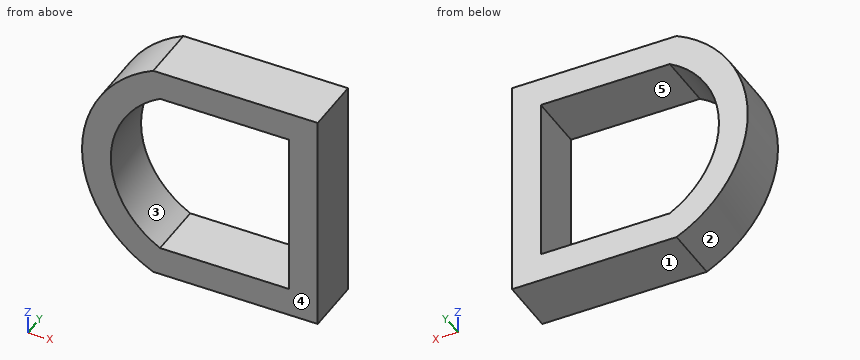
Autodesk Inventor part; units mm, degrees
ref_plane "YZ Plane" through (0, 0, 0) normal (1, 0, 0) x (0, 1, 0)
ref_plane "XZ Plane" through (0, 0, 0) normal (0, 1, 0) x (-1, 0, 0)
ref_plane "XY Plane" through (0, 0, 0) normal (0, 0, 1) x (1, 0, 0)
sketch "Sketch1" plane through (0, 0, 0) normal (0, 1, 0) x (-1, 0, 0)
  line L0 (53.122, 125.6518) -> (38.898, 125.6518)
  line L1 (38.898, 125.6518) -> (38.898, 107.3638)
  line L2 (38.898, 107.3638) -> (53.122, 107.3638)
  arc A0 (53.122, 107.3638) -> (53.122, 125.6518) centre (48.1382, 116.5078) ccw
  line L3 (51.0559, 55.1199) -> (37.0859, 55.1199)
  line L4 (37.0859, 55.1199) -> (37.0859, 37.0859)
  line L5 (37.0859, 37.0859) -> (51.0559, 37.0859)
  arc A1 (51.0559, 37.0859) -> (51.0559, 55.1199) centre (39.6314, 46.1029) ccw
  line L6 (61.7452, 17.3999) -> (47.7752, 17.3999)
  line L7 (47.7752, 17.3999) -> (47.7752, -0.6341)
  line L8 (47.7752, -0.6341) -> (61.7452, -0.6341)
  arc A2 (61.7452, -0.6341) -> (61.7452, 17.3999) centre (49.459, 8.3829) ccw
  line L9 (89.1373, 73.7746) -> (75.1673, 73.7746)
  line L10 (75.1673, 73.7746) -> (75.1673, 55.7406)
  line L11 (75.1673, 55.7406) -> (89.1373, 55.7406)
  arc A3 (89.1373, 55.7406) -> (89.1373, 73.7746) centre (83.9272, 64.7576) ccw
  line L12 (52.5031, 58.2949) -> (33.9109, 58.2949)
  line L13 (33.9109, 58.2949) -> (33.9109, 33.9109)
  line L14 (33.9109, 33.9109) -> (52.5031, 33.9109)
  arc A4 (52.5031, 33.9109) -> (52.5031, 58.2949) centre (39.6314, 46.1029) ccw
  line L15 (53.8743, 128.8268) -> (35.723, 128.8268)
  line L16 (35.723, 128.8268) -> (35.723, 104.1888)
  line L17 (35.723, 104.1888) -> (53.8743, 104.1888)
  arc A5 (53.8743, 104.1888) -> (53.8743, 128.8268) centre (48.1382, 116.5078) ccw
  line L18 (63.26, 20.5749) -> (44.6002, 20.5749)
  line L19 (44.6002, 20.5749) -> (44.6002, -3.8091)
  line L20 (44.6002, -3.8091) -> (63.26, -3.8091)
  arc A6 (63.26, -3.8091) -> (63.26, 20.5749) centre (49.459, 8.3829) ccw
  line L21 (89.9285, 52.5656) -> (71.9923, 52.5656)
  line L22 (71.9923, 52.5656) -> (71.9923, 76.9496)
  line L23 (71.9923, 76.9496) -> (89.9285, 76.9496)
  arc A7 (89.9285, 52.5656) -> (89.9285, 76.9496) centre (83.9272, 64.7576) ccw
  point P0 (0, 0)
  dimension "d0" = 10.414
  dimension "d1" = 14.224
  dimension "d2" = 18.288
  dimension "d3" = 14.5542
  dimension "d4" = 13.97
  dimension "d5" = 18.034
  dimension "d6" = 15.24
  dimension "d7" = 13.97
  dimension "d8" = 18.034
  dimension "d10" = 13.97
  dimension "d11" = 18.034
  dimension "d13" = 3.175
  dimension "d14" = 3.175
  dimension "d15" = 3.175
  dimension "d19" = 10.414
  dimension "d20" = 3.175
extrude "Extrusion2" add sketch "Sketch1" along normal blind 6.35 contours A5 L17 L16 L15
properties part number "truck_sizings"
The listing builds one solid part. Answer for the finished solid, in the listing's coordinates (mm). Face numbers are marked on the shaded views. A direction names the side the tool comes from. Round coordinates to 2 decimals unless told otherwise and drop trailing zeros. Write each loop counter-clockwise with the first axis right and the second up, starting at its lowest first coordinate (ties: lowest second). Pieces come first, ordered by that corner, then holes. Notation, with made-up numbers: (18, 85) - (27, 85) arc R5 ccw to (27, 92) - close; hole circle Ø3 at (18.5, -10). An arc over 180 degrees is marked (long way). Use a Markdown table: item, result. Add a question column.
1. Consider line 1 (Z direction, x = -44.75, y = 2); line 2 (X direction, y = 2.5, z = 113.75); line 3 (X direction, y = 1.75, z = 109.25). Determine where each line is inside the solid, lowest interval first.
2. For a pull along Z with two mould halves and no side action, classify the marked faces 1, 2 and 3 as +Z half, -Z half, draft (parallel to the pull), parting line (faces both ways), or undercut.
3. A tool of negligible diameter and unlimited length cuts with its end or side. For the marked faces 4 and 5, from which of +Z, -Z, +X, -X, +Y, -Y can it reach the whole face along a straight path? Write none if from no direction.
4. The part is cut by section D-D (x = -60). Write down the section's boundary in (y, z), and give its area (3 significant figures).
5. The part is cut by section A-A (x = -41.75). Write down the section's boundary in (y, z), and give its area (3 significant figures).
6. The part is cut by section C-C (z = 120). Write down the section's boundary in (x, y).
7. The part is cut by section B-B (y = 2.75). Write down the section's boundary in (x, z), and give its area (3 significant figures).
Reported:
| question | item | result |
|---|---|---|
| 1 | line 1 | 104.19 to 107.36, 125.65 to 128.83 |
| 1 | line 2 | -61.44 to -58.18, -38.9 to -35.72 |
| 1 | line 3 | -59.63 to -55.61, -38.9 to -35.72 |
| 2 | face 1 | -Z half |
| 2 | face 2 | parting line |
| 2 | face 3 | undercut |
| 3 | face 4 | +Z, -Z, +X, -X, -Y |
| 3 | face 5 | +Y, -Y |
| 4 | outline | (0, 109.88) - (6.35, 109.88) - (6.35, 123.14) - (0, 123.14) - close |
| 4 | area | 84.2 mm^2 |
| 5 | outline | (0, 104.19) - (6.35, 104.19) - (6.35, 107.36) - (0, 107.36) - close; (0, 125.65) - (6.35, 125.65) - (6.35, 128.83) - (0, 128.83) - close |
| 5 | area | 40.3 mm^2 |
| 6 | outline | (-61.27, 0) - (-57.95, 0) - (-57.95, 6.35) - (-61.27, 6.35) - close; (-38.9, 0) - (-35.72, 0) - (-35.72, 6.35) - (-38.9, 6.35) - close |
| 7 | outline | (-53.87, 104.19) - (-35.72, 104.19) - (-35.72, 128.83) - (-53.87, 128.83) arc R13.59 ccw to start; hole (-53.12, 107.36) - (-38.9, 107.36) - (-38.9, 125.65) - (-53.12, 125.65) arc R10.41 ccw to start |
| 7 | area | 255 mm^2 |
